from build123d import *

# Parameters (mm, degrees)
F0_R           = 14
F0_W           = 178
F0_H           = 24
F1_DEPTH       = 25
F2_DEPTH       = 40
F3_DEPTH       = 68
F4_R           = 20
F6_D           = 10
F6_CBORE_D     = 20
F6_CBORE_DEPTH = 10


with BuildPart() as f1:
    # F0 (on Front) → F1 (new body)
    with BuildSketch(Plane.XZ):
        with BuildLine():
            ThreePointArc((-29.54449, 5.207985), (-2.613934, -29.885906), (30, 0))
            ThreePointArc((30, 0), (29.885906, 2.613934), (29.54449, 5.207985))
            ThreePointArc((29.54449, 5.207985), (0, 30), (-29.54449, 5.207985))
        make_face()
        Circle(F0_R, mode=Mode.SUBTRACT)
        with BuildLine():
            ThreePointArc((29.54449, 5.207985), (29.885906, 2.613934), (30, 0))
            ThreePointArc((30, 0), (-2.613934, -29.885906), (-29.54449, 5.207985))
            ThreePointArc((-29.54449, 5.207985), (-45.525876, -23.445808), (-75.828036, -36.024509))
            ThreePointArc((-75.828036, -36.024509), (-85.188045, -40.397722), (-89, -50))
            Line((-89, -50), (89, -50))
            ThreePointArc((89, -50), (85.188045, -40.397722), (75.828036, -36.024509))
            ThreePointArc((75.828036, -36.024509), (45.525876, -23.445808), (29.54449, 5.207985))
        make_face()
        with Locations((0, -62)):
            Rectangle(F0_W, F0_H)
    extrude(amount=F1_DEPTH)

    # F0 (on Front) → F2 (join)
    with BuildSketch(Plane.XZ):
        with BuildLine():
            ThreePointArc((-29.54449, 5.207985), (-2.613934, -29.885906), (30, 0))
            ThreePointArc((30, 0), (29.885906, 2.613934), (29.54449, 5.207985))
            ThreePointArc((29.54449, 5.207985), (0, 30), (-29.54449, 5.207985))
        make_face()
        Circle(F0_R, mode=Mode.SUBTRACT)
    extrude(amount=F2_DEPTH)

    # F0 (on Front) → F3 (join)
    with BuildSketch(Plane.XZ):
        with Locations((0, -62)):
            Rectangle(F0_W, F0_H)
    extrude(amount=F3_DEPTH)

    # F4
    f4_edges = [f1.edges().sort_by_distance(p)[0] for p in [
        (-89, -68, -62),
        (89, -68, -62),
    ]]
    fillet(f4_edges, radius=F4_R)

    # F6 (through all)
    with Locations(Plane.XY.offset(-50)):
        with Locations((-65, -48.848685), (65, -48.848685)):
            CounterBoreHole(F6_D / 2, F6_CBORE_D / 2, F6_CBORE_DEPTH)


solid = f1.part
Here's how the part is built. I have some questions about the finished solid (model axes, mm). A direction names the side the tool comes from. Coordinates: 2 decimals unless noted, no trailing zeros. Order: outer loops, then holes, each group sorted by start corner. A loop starts at its lowest first (then second) coordinate and runs counter-clockwise, first axis right, second up. Notation, with made-up numbers: (48.5, -30.5) - (107.5, -30.5) arc R32 ccw to (107.5, 1.5) - close; hole circle Ø10 at (4, 68.25). An arc over 180 degrees is marked (long way). Use CSV: the item, a comma, the result in double quotes. Start each with the question number.
1. Suppose I cut it at A-A on x = 0. List the corners of the cut face in (y, z) for me.
2. Suppose I cut it at C-C on x = 73. List the corners of the cut face in (y, z) for me.
3. I'm going to push flat-ended pins straight in: pin 1 (22 mm diameter, centred on x = 63.5, y = -48.5, fed in from +Z); pin 2 (6 mm diameter, centred on x = -30, z = -40.5, fed in from -Y); pin 3 (12 mm diameter, centred on y = -28, z = -42.5, fed in from +X); pin 4 (9 mm diameter, centred on x = 65, y = -48.85, fed in from -Z). Where does each tip first touch, or does it pass through?
4. Suppose I cut it at B-B on y = -9. List the corners of the cut face in (x, z) for me, then the cut area to 3 significant figures.
5. For faces 1 (the face through (29.89, -32.39, 2.58)), 2 (the face through (13, -40, -6)), 3 (the face through (55.01, -48.41, -54.93)), 4 (the face through (-45.178, -12.325, -23.133)), 5 (the face through (-1, -25, -34)), which set-ups out of +Z, -Z, +X, -X, +Y, -Y let a thin tool reach every point of the face, with its end or its side?
6. Suppose I cut it at D-D on z = 20.5. List the corners of the cut face in (x, y) for me.
7. If we mould it in two halves opening along Y, with no side actions, what happens to faces 6 (the face through (-70, -51, -60)), 7 (the face through (-82.986, -62.297, -61.832)), 8 (the face through (-1, -46, -50)), 9 (the face through (-74.99, -48.41, -54.93))? For each: +Y half, -Y half, draft (parallel to the pull), parting line (faces both ways), or undercut.
8. Please list where these lines run through material, in increasing order: line 1 (Z direction, x = 0, y = -27); line 2 (Y direction, x = 65, z = -54.75); line 3 (Y direction, x = -65, z = -64.25). Write a range as from..to.
Output:
1,outline,"(-68, -74) - (0, -74) - (0, -14) - (-40, -14) - (-40, -30) - (-25, -30) - (-25, -50) - (-68, -50) - close; (-40, 14) - (0, 14) - (0, 30) - (-40, 30) - close"
2,outline,"(-67.6, -74) - (0, -74) - (0, -35.78) - (-25, -35.78) - (-25, -50) - (-42.85, -50) - (-42.85, -60) - (-54.85, -60) - (-54.85, -50) - (-67.6, -50) - close"
3,pin 1,"stops at z = -50"
3,pin 2,"stops at y = -25"
3,pin 3,"stops at x = 88.81"
3,pin 4,"passes through"
4,outline,"(-89, -74) - (89, -74) - (89, -50) arc R14 ccw to (75.83, -36.02) arc R50 cw to (29.54, 5.21) arc R30 ccw to (-29.54, 5.21) arc R50 cw to (-75.83, -36.02) arc R14 ccw to (-89, -50) - close; hole circle Ø28 at (0, 0)"
4,area,"10,600 mm2"
5,face 1,"+Z, +X, -Y"
5,face 2,"+Z, +X, -X, -Y"
5,face 3,"+Z"
5,face 4,"+Z, -X, +Y, -Y"
5,face 5,"-Y"
6,outline,"(-21.9, -40) - (21.9, -40) - (21.9, 0) - (-21.9, 0) - close"
7,face 6,"undercut"
7,face 7,"-Y half"
7,face 8,"draft"
7,face 9,"undercut"
8,line 1,"z = -74..-50, -30..-14, 14..30"
8,line 2,"y = -68..-58.85, -38.85..0"
8,line 3,"y = -68..-53.85, -43.85..0"
